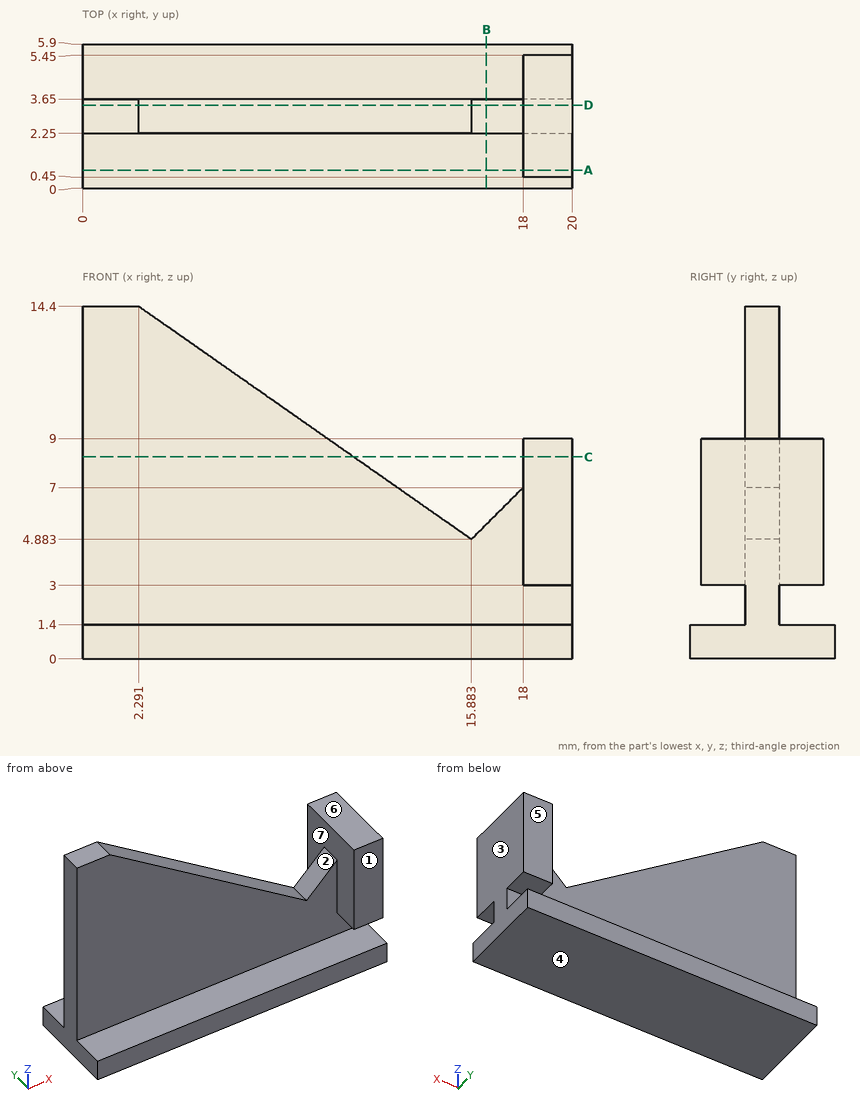
The figure shows three views and two pictorial views of one solid part (mm, origin at its lowest corner). Answer the questions. A direction names the side the tool comes from. Give positions to 0.01 mm unless a question says otherwise; leave off trailing zeros. Order: outer loops, then holes, each group sorted by start corner. A loop starts at its lowest first (then second) coordinate and runs counter-clockwise, first axis right, second up. Notation, with made-up numbers: (1, 3.5) -> (35, 3.5) arc R29 cw to (35, 24.5) -> close; hole circle Ø8 at (51.25, 2). An arc over 180 degrees is marked (long way). Answer as CSV lines item,"result". Start each with the question number.
(1) Section D-D, the plane y = 3.4 is taken. Write down the section's boundary in (x, z), plus the area to 3 significant figures.
(2) Which of the six approach directions +Z, -Z, +X, -X, +Y, -Y give full straight-line access (tool end or side, diameter ignored) to the marked faces 4, 5, 6 and 7?
(3) Section A-A, the plane y = 0.75 is taken. Write down the section's boundary in (x, z).
(4) Each of these flat-tipped pins is pushed along its axis until it touches: pin 1 Ø2 at (x, z) = (18.5, 6.5) entering from -Y; pin 2 Ø4 at (x, z) = (14.5, 9.5) entering from +Y; pin 3 Ø2 at (x, y) = (9.5, 3.5) entering from +Z; pin 4 Ø3 at (x, y) = (3.5, 5) entering from +Z. Where does it stop, or does it pass through?
(5) Section C-C, the plane z = 8.25 is taken. Write down the section's boundary in (x, y).
(6) Section B-B, the plane x = 16.5 is taken. Write down the section's boundary in (y, z), plus the area to 3 significant figures.
(7) For a pull along X with two mould halves and no side action, classify the marked faces 1, 2 and 3 as released by +X, released by -X, zero draft, split by the parting line, or undercut.
(8) Consider line 1 along Z through (x, y) = (19, 4.05); line 2 along Y through (x, z) = (9.5, 8); line 3 along Y through (x, z) = (19, 8.5). Determine where each line is inside the solid, lowest interval first.
Entries:
1,outline,"(0, 0) -> (20, 0) -> (20, 9) -> (18, 9) -> (18, 7) -> (15.88, 4.88) -> (2.29, 14.4) -> (0, 14.4) -> close"
1,area,"195 mm²"
2,face 4,"-Z, +X, -X, +Y, -Y"
2,face 5,"+Z, +X, -X, +Y"
2,face 6,"+Z, +X, +Y, -Y"
2,face 7,"+Z"
3,outline,"(0, 0) -> (20, 0) -> (20, 1.4) -> (0, 1.4) -> close; (18, 3) -> (20, 3) -> (20, 9) -> (18, 9) -> close"
4,pin 1,"y = 0.45"
4,pin 2,"through"
4,pin 3,"z = 10.05"
4,pin 4,"z = 14.01"
5,outline,"(0, 2.25) -> (11.07, 2.25) -> (11.07, 3.65) -> (0, 3.65) -> close; (18, 0.45) -> (20, 0.45) -> (20, 5.45) -> (18, 5.45) -> close"
6,outline,"(0, 0) -> (5.9, 0) -> (5.9, 1.4) -> (3.65, 1.4) -> (3.65, 5.5) -> (2.25, 5.5) -> (2.25, 1.4) -> (0, 1.4) -> close"
6,area,"14.0 mm²"
7,face 1,"zero draft"
7,face 2,"undercut"
7,face 3,"released by +X"
8,line 1,"0 to 1.4, 3 to 9"
8,line 2,"2.25 to 3.65"
8,line 3,"0.45 to 5.45"
